Could you check a few things on this drawing? It's one solid part, dimensions in mm from its lowest x, y, z. A direction names the side the tool comes from. Round coordinates to 2 decimals unless told otherwise and drop trailing zeros. Loops run counter-clockwise (first coordinate to the right, second up) from the corner with the lowest first, then second, coordinate; pieces in that order, holes last. Notation, with made-up numbers: (54, -37) -> (108, -37) arc R26 ccw to (108, -7) -> close; hole circle Ø11 at (42, -18). An arc over 180 degrees is marked (long way). Put each result on its own line as item: value. Start each with the question number.
1. Which directions (+Z, -Z, +X, -X, +Y, -Y) give clear straight access to the entire face, cutting with the end or side of a thin tool? Please do the marked faces 1 and 2.
2. Imagine slicing it at A-A, the plane y = 40. Please give me the cut outline in (x, z).
3. Imagine slicing it at D-D, the plane z = 19.5. Please give me the cut outline in (x, y), and give its area (3 significant figures).
4. Imagine slicing it at B-B, the plane z = 32. Please give me the cut outline in (x, y) (3 decimals).
5. I'm going to push flat-ended pins straight in: P1, Ø2, axis at x = 20, y = 57, coming from the +Z side; P2, Ø2.5, axis at x = 38, z = 15.5, coming from the +Y side; P3, Ø6, axis at y = 53, z = 19, coming from the +X side (1 decimal); P4, Ø4, axis at y = 9, z = 20, coming from the -X side. Where does each tip first touch, or does it pass through?
6. Imagine slicing it at C-C, the plane y = 11.5. Please give me the cut outline in (x, z), and give its area (3 significant figures).
7. I need wall thicknesses on line 1 (X direction, y = 40, z = 1.4); line 2 (X direction, y = 38.5, z = 18); line 3 (Z direction, x = 7.5, y = 26.5). Which ranges of each line are inside material? Lowest first, please. Write a range as [from, to].
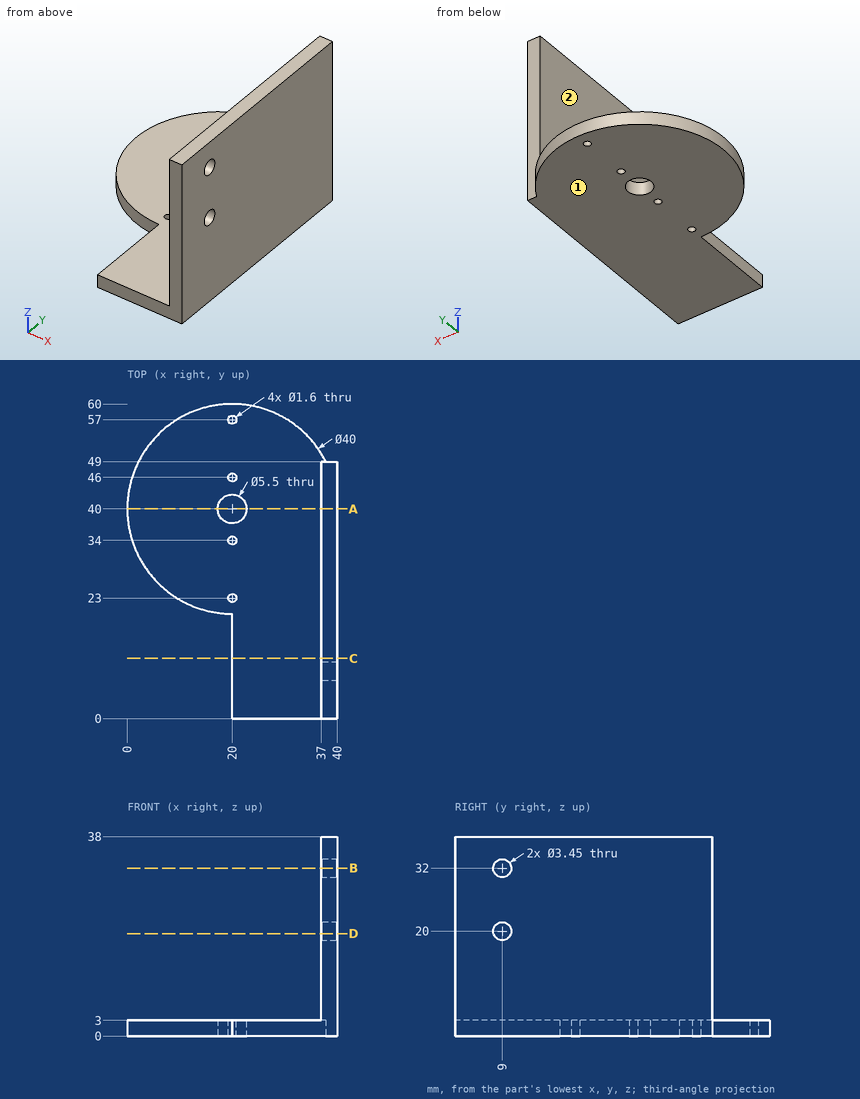
Entries:
1. face 1: -Z, +X, -X, +Y, -Y
1. face 2: +Z, -X, +Y, -Y
2. outline: (0, 0) -> (17.25, 0) -> (17.25, 3) -> (0, 3) -> close; (22.75, 0) -> (40, 0) -> (40, 38) -> (37, 38) -> (37, 3) -> (22.75, 3) -> close
3. outline: (37, 0) -> (40, 0) -> (40, 7.35) -> (37, 7.35) -> close; (37, 10.65) -> (40, 10.65) -> (40, 49) -> (37, 49) -> close
3. area: 137 mm^2
4. outline: (37, 0) -> (40, 0) -> (40, 7.275) -> (37, 7.275) -> close; (37, 10.725) -> (40, 10.725) -> (40, 49) -> (37, 49) -> close
5. P1: z = 3
5. P2: y = 49
5. P3: through
5. P4: x = 37
6. outline: (20, 0) -> (40, 0) -> (40, 38) -> (37, 38) -> (37, 3) -> (20, 3) -> close
6. area: 165 mm^2
7. line 1: [0, 17.25], [22.75, 40]
7. line 2: [37, 40]
7. line 3: [0, 3]
